For this review, take the finished solid that the model builds, in its own axes (mm). Face numbers are marked on the shaded views. A direction names the side the tool comes from. Round coordinates to 2 decimals unless told otherwise and drop trailing zeros. Order: outer loops, then holes, each group sorted by start corner. A loop starts at its lowest first (then second) coordinate and runs counter-clockwise, first axis right, second up.
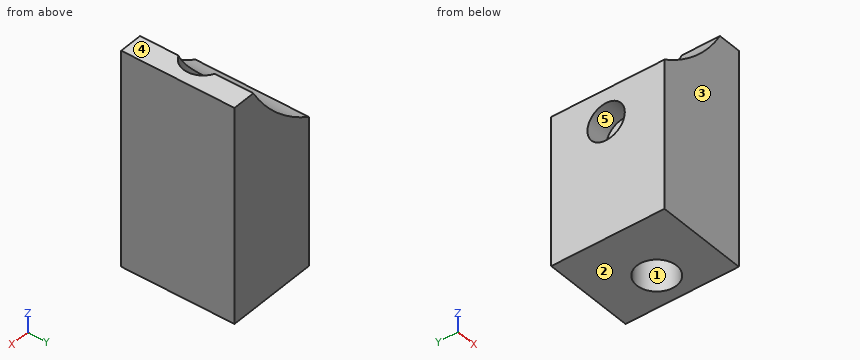
```python
from build123d import *

# Parameters (mm, degrees)
SKETCH_W        = 7.9
SKETCH_H        = 9.7
PAD_DEPTH       = 26
SKETCH002_R     = 1.7
POCKET001_DEPTH = 26
SKETCH003_R     = 4
SKETCH003_R_2   = 15
POCKET002_DEPTH = 10
SKETCH004_R     = 1.7
POCKET003_DEPTH = 2
SKETCH005_W     = 2
SKETCH005_H     = 7.483315
POCKET_DEPTH    = 10
SKETCH006_R     = 1.6
POCKET004_DEPTH = 2


with BuildPart() as part:
    # Sketch → Pad (new body)
    with BuildSketch(Plane.XY):
        with Locations((-29.043821, 17.932895)):
            Rectangle(SKETCH_W, SKETCH_H)
    extrude(amount=PAD_DEPTH)

    # Sketch002 → Pocket001 (cut)
    with BuildSketch(Plane.XY.offset(26)):
        with Locations((-27.793821, 17.932895)):
            Circle(SKETCH002_R)
    extrude(amount=-POCKET001_DEPTH, mode=Mode.SUBTRACT)

    # Sketch003 → Pocket002 (cut)
    with BuildSketch(Plane.XZ.offset(-13.082895)):
        with Locations((-19.856678, 26)):
            Circle(SKETCH003_R)
        with Locations((-40.093821, 26)):
            Circle(SKETCH003_R_2)
    extrude(amount=-POCKET002_DEPTH, mode=Mode.SUBTRACT)

    # Sketch004 → Pocket003 (cut)
    with BuildSketch(Plane(origin=(0, 22.782895, 0), x_dir=(-1, 0, 0), z_dir=(0, 1, 0))):
        with Locations((-19.682895, 11)):
            Circle(SKETCH004_R)
    extrude(amount=-POCKET003_DEPTH, mode=Mode.SUBTRACT)

    # Sketch005 → Pocket (cut)
    with BuildSketch(Plane.XZ.offset(-13.082895)):
        with Locations((-26.093821, 22.258342)):
            Rectangle(SKETCH005_W, SKETCH005_H)
    extrude(amount=-POCKET_DEPTH, mode=Mode.SUBTRACT)

    # Sketch006 → Pocket004 (cut)
    with BuildSketch(Plane(origin=(-32.993821, 0, 0), x_dir=(0, -1, 0), z_dir=(-1, 0, 0))):
        with Locations((-18.082895, 10)):
            Circle(SKETCH006_R)
    extrude(amount=-POCKET004_DEPTH, mode=Mode.SUBTRACT)


solid = part.part
```
Q1. Take a section at C-C, the plane z = 10. State the section outline as (x, y) points.
Q2. Mouldability with a two-part tool opening along Y and no side actions: class the marked faces 1, 2 and 3 as +Y half, -Y half, draft (parallel to the pull), parting line (faces both ways), or undercut.
Q3. Wall thickness on line 1 (X direction, y = 18, z = 11.25); line 2 (X direction, y = 17, z = 4.75); line 3 (Z direction, x = -31.5, y = 18.25): over which ranges is each line inside the solid? List them lowest first.
Q4. Take a section at B-B, the plane x = -27.5. State the section outline as (y, z) points, plus the area to 3 significant figures.
Q5. Tool access review of the marked faces 4 and 5: name each direction out of +Z, -Z, +X, -X, +Y, -Y from which nothing blocks a thin tool from reaching the whole face with its end or side.
Q6. Take a section at D-D, the plane y = 14.25. State the section outline as (x, z) points, plus the area to 3 significant figures.
Q7. Clearance check with flat-ended pins moving along their axes: pin 1 (2 mm diameter, centred on x = -30, y = 15.5, fed in from +Z); pin 2 (1 mm diameter, centred on y = 18, z = 10.5, fed in from -X); pin 3 (2 mm diameter, centred on y = 16, z = 14, fed in from -X). State where each tip first meets the part, or that it passes through.
Q8. Take a section at A-A, the plane y = 19. State the section outline as (x, z) points, plus the area to 3 significant figures.
Working result:
1. outline: (-32.99, 13.08) - (-25.09, 13.08) - (-25.09, 22.78) - (-32.99, 22.78) - (-32.99, 19.68) - (-30.99, 19.68) - (-30.99, 16.48) - (-32.99, 16.48) - close; hole circle Ø3.4 at (-27.79, 17.93)
2. face 1: undercut
2. face 2: draft
2. face 3: -Y half
3. line 1: x = -30.99 to -29.49, -26.1 to -25.09
3. line 2: x = -32.99 to -29.21, -26.37 to -25.09
3. line 3: z = 0 to 8.41, 11.59 to 13.71
4. outline: (13.08, 0) - (16.26, 0) - (16.26, 17.85) - (13.08, 17.85) - close; (19.61, 0) - (22.78, 0) - (22.78, 17.85) - (19.61, 17.85) - close
4. area: 113 mm2
5. face 4: +Z, +X, -X, +Y, -Y
5. face 5: -X
6. outline: (-32.99, 0) - (-25.09, 0) - (-25.09, 18.52) - (-27.09, 18.52) arc R15 cw to (-32.99, 12.79) - close
6. area: 126 mm2
7. pin 1: stops at z = 15.9
7. pin 2: stops at x = -30.99
7. pin 3: stops at x = -32.61
8. outline: (-32.99, 0) - (-29.12, 0) - (-29.12, 15.78) arc R15 cw to (-32.99, 12.79) - (-32.99, 11.31) - (-30.99, 11.31) - (-30.99, 8.69) - (-32.99, 8.69) - close; (-26.47, 0) - (-25.09, 0) - (-25.09, 18.52) - (-26.47, 18.52) - close
8. area: 75.0 mm2
